from build123d import *

# Parameters (mm, degrees)
SKETCH1_R           = 1.2
SKETCH1_R_2         = 27.25
SKETCH1_R_3         = 25.5
BOSS_EXTRUDE1_DEPTH = 2
SKETCH2_R           = 25.5
BOSS_EXTRUDE3_DEPTH = 1
SKETCH3_R           = 1.5
BOSS_EXTRUDE4_DEPTH = 4
CHAMFER1_SIZE       = 1
CHAMFER2_SIZE       = 1
CUT_EXTRUDE1_DEPTH  = 2
SKETCH5_R           = 0.6
BOSS_EXTRUDE5_DEPTH = 0.4
CHAMFER3_SIZE       = 0.5
FILLET1_R           = 0.5


with BuildPart() as part:
    # Sketch1 → Boss-Extrude1 (new body)
    # profile 1 of 5: a face of its own
    with BuildSketch(Plane(origin=(0, 0, 0), x_dir=(1, 0, 0), z_dir=(0, 1, 0))):
        with BuildLine():
            ThreePointArc((-28.722813233, 16.1), (-29.965874009, 13.647578353), (-31, 11.1))
            Line((-31, 11.1), (-24.886793687, 11.1))
            ThreePointArc((-24.886793687, 11.1), (-20.899896158, 17.485904054), (-15.317841085, 22.537219094))
            ThreePointArc((-15.317841085, 22.537219094), (-21.77967806, 18.817477861), (-28.722813233, 16.1))
        make_face()
        with Locations(Location((-27.128197522, 13.481505135, 0), (0, 0, 270))):
            Circle(SKETCH1_R, mode=Mode.SUBTRACT)
    # profile 2 of 5: a face of its own
    with BuildSketch(Plane(origin=(0, 0, 0), x_dir=(1, 0, 0), z_dir=(0, 1, 0))):
        with BuildLine():
            ThreePointArc((-15.317841085, -22.537219094), (-20.899896158, -17.485904054), (-24.886793687, -11.1))
            Line((-24.886793687, -11.1), (-31, -11.1))
            ThreePointArc((-31, -11.1), (-29.965874009, -13.647578353), (-28.722813233, -16.1))
            ThreePointArc((-28.722813233, -16.1), (-21.77967806, -18.817477861), (-15.317841085, -22.537219094))
        make_face()
        with Locations(Location((-27.128197522, -13.718494865, 0), (0, 0, 270))):
            Circle(SKETCH1_R, mode=Mode.SUBTRACT)
    # profile 3 of 5: a face of its own
    with BuildSketch(Plane(origin=(0, 0, 0), x_dir=(1, 0, 0), z_dir=(0, 1, 0))):
        Circle(SKETCH1_R_2)
        with Locations(Location((0, 0, 0), (0, 0, 270))):
            Circle(SKETCH1_R_3, mode=Mode.SUBTRACT)
    # profile 4 of 5: a face of its own
    with BuildSketch(Plane(origin=(0, 0, 0), x_dir=(1, 0, 0), z_dir=(0, 1, 0))):
        with BuildLine():
            ThreePointArc((24.886793687, -11.1), (20.899896158, -17.485904054), (15.317841085, -22.537219094))
            ThreePointArc((15.317841085, -22.537219094), (21.77967806, -18.817477861), (28.722813233, -16.1))
            ThreePointArc((28.722813233, -16.1), (29.965874009, -13.647578353), (31, -11.1))
            Line((31, -11.1), (24.886793687, -11.1))
        make_face()
        with Locations(Location((26.871802478, -13.718494865, 0), (0, 0, 270))):
            Circle(SKETCH1_R, mode=Mode.SUBTRACT)
    # profile 5 of 5: a face of its own
    with BuildSketch(Plane(origin=(0, 0, 0), x_dir=(1, 0, 0), z_dir=(0, 1, 0))):
        with BuildLine():
            ThreePointArc((28.722813233, 16.1), (21.77967806, 18.817477861), (15.317841085, 22.537219094))
            ThreePointArc((15.317841085, 22.537219094), (20.899896158, 17.485904054), (24.886793687, 11.1))
            Line((24.886793687, 11.1), (31, 11.1))
            ThreePointArc((31, 11.1), (29.965874009, 13.647578353), (28.722813233, 16.1))
        make_face()
        with Locations(Location((26.871802478, 13.481505135, 0), (0, 0, 270))):
            Circle(SKETCH1_R, mode=Mode.SUBTRACT)
    extrude(amount=BOSS_EXTRUDE1_DEPTH)

    # Sketch2 → Boss-Extrude3 (add)
    with BuildSketch(Plane.XZ):
        with Locations(Location((0, 0, 0), (0, 0, 270))):
            Circle(SKETCH2_R)
    extrude(amount=-BOSS_EXTRUDE3_DEPTH)

    # Sketch3 → Boss-Extrude4 (add)
    with BuildSketch(Plane.XZ):
        with Locations(Location((-27.128197522, 13.718494865, 0), (0, 0, 270))):
            Circle(SKETCH3_R)
        with Locations(Location((26.871802478, 13.718494865, 0), (0, 0, 270))):
            Circle(SKETCH3_R)
        with Locations(Location((26.871802478, -13.481505135, 0), (0, 0, 270))):
            Circle(SKETCH3_R)
        with Locations(Location((-27.128197522, -13.481505135, 0), (0, 0, 270))):
            Circle(SKETCH3_R)
    extrude(amount=-BOSS_EXTRUDE4_DEPTH)

    # Chamfer1
    chamfer1_edges = [part.edges().sort_by_distance(p)[0] for p in [
        (0, 0, -27.25),
        (21.77967806, 0, -18.817477861),
        (29.965874009, 0, -13.647578353),
        (27.943396843, 0, -11.1),
        (27.25, 0, 0),
        (27.943396843, 0, 11.1),
        (29.965874009, 0, 13.647578353),
        (21.77967806, 0, 18.817477861),
        (0, 0, 27.25),
        (-21.77967806, 0, 18.817477861),
        (-29.965874009, 0, 13.647578353),
        (-27.943396843, 0, 11.1),
        (-27.25, 0, 0),
        (-27.943396843, 0, -11.1),
        (-29.965874009, 0, -13.647578353),
        (-21.77967806, 0, -18.817477861),
    ]]
    chamfer(chamfer1_edges, length=CHAMFER1_SIZE)

    # Chamfer2
    chamfer2_edges = [part.edges().sort_by_distance(p)[0] for p in [
        (0, 1, -25.5),
    ]]
    chamfer(chamfer2_edges, length=CHAMFER2_SIZE - 0.0001)  # a hair under: the kernel refuses the full size

    # Sketch4 → Cut-Extrude1 (cut)
    with BuildSketch(Plane(origin=(0, 1, 0), x_dir=(1, 0, 0), z_dir=(0, 1, 0))):
        Polygon((-7.518498865, -7.181133816), (-1.722943541, -8.734046717), (-2.551163755, -11.825009557), (-8.346719079, -10.272096656), align=None)
    extrude(amount=-CUT_EXTRUDE1_DEPTH, mode=Mode.SUBTRACT)

    # Sketch5 → Boss-Extrude5 (add)
    with BuildSketch(Plane(origin=(0, 1, 0), x_dir=(1, 0, 0), z_dir=(0, 1, 0))):
        with Locations(Location((1.460899698, -12.082012325, 0), (0, 0, 90))):
            Circle(SKETCH5_R)
        with Locations(Location((-9.793498218, -4.821776272, 0), (0, 0, 90))):
            Circle(SKETCH5_R)
    extrude(amount=BOSS_EXTRUDE5_DEPTH)

    # Chamfer3
    chamfer3_edges = [part.edges().sort_by_distance(p)[0] for p in [
        (-7.932608972, 1, 8.726615236),
        (-5.448941417, 1, 11.048553106),
        (-2.137053648, 1, 10.279528137),
        (-4.620721203, 1, 7.957590266),
    ]]
    chamfer(chamfer3_edges, length=CHAMFER3_SIZE)

    # Fillet1
    fillet1_edges = [part.edges().sort_by_distance(p)[0] for p in [
        (-27.128197522, 4, 15.218494865),
        (26.871802478, 4, 15.218494865),
        (26.871802478, 4, -11.981505135),
        (-27.128197522, 4, -11.981505135),
    ]]
    fillet(fillet1_edges, radius=FILLET1_R)


solid = part.part
Source: CAD feature listing. Evaluate the final solid. Frame: model axes, mm. A direction names the side the tool comes from. Coordinates: 2 decimals unless noted, no trailing zeros. Write each question's results on one line, items separated by ' | '. Start each with the question number.
1. Pin query (flat end, axial travel): pin 1 (1.1 mm diameter, centred on x = -27, y = 1.5, fed in from +Z); pin 2 (1.3 mm diameter, centred on x = -10, z = 5, fed in from +Y); pin 3 (1.5 mm diameter, centred on y = 0.5, z = -14, fed in from -X); pin 4 (1 mm diameter, centred on y = 3, z = -18, fed in from +X). Return the tip coordinate at first contact, or that it passes through.
2. Reachability of faces 4 (the face through (21.874, 1.493, -18.772)), 5 (the face through (-4.604, 0.746, 7.707)) from +Z, -Z, +X, -X, +Y, -Y: full face, straight path, thin tool, end or side. Return the list, or none.
3. Material intervals for L1, parallel to Y at x = 17, z = -11; L2, parallel to Y at x = 18, z = 19; L3, parallel to Z at x = -10, y = 1.3, sorted ascending.
4. Draft query along X for faces 1 (the face through (-29.279, 0.507, 13.955)), 2 (the face through (26.42, 0.17, 0.18)), 3 (the face through (0, 1, 0)). Return one class per face: +X half, -X half, draft (parallel to the pull), parting line (faces both ways), or undercut.
Solution:
1) pin 1: z = 16.86 | pin 2: y = 1.4 | pin 3: x = -30.06 | pin 4: through
2) face 4: -Z, +X, +Y, -Y | face 5: +Y
3) L1: 0 to 1 | L2: 0 to 2 | L3: -25.35 to -22.69, 4.26 to 5.39, 22.69 to 25.35
4) face 1: -X half | face 2: +X half | face 3: undercut
